Check sheet for the modelled part. Datum: model origin and axes. Units: mm. Face numbers are marked on the shaded views. A direction names the side the tool comes from. Round coordinates to 2 decimals unless told otherwise and drop trailing zeros. Write each loop counter-clockwise with the first axis right and the second up, starting at its lowest first coordinate (ties: lowest second). Pieces come first, ordered by that corner, then holes. Notation, with made-up numbers: (52, -28.75) - (100, -28.75) arc R23 cw to (100, -4.75) - close; hole circle Ø8 at (51, 10.5). An arc over 180 degrees is marked (long way). Answer as a JSON object with one key per item and string values. Group by question number.
Item 1: Thickness scan on line 1 (Z direction, x = 4.5, y = -15); line 2 (X direction, y = -6, z = -3.75); line 3 (Z direction, x = 4.25, y = -19). Record the ranges inside material, lowest first.
Item 2: Release check for a two-part mould opening along X. For the marked faces 5, 6 and 7 record: pulls with the +X half, pulls with the -X half, needs draft (parallel to the pull), parting line crosses it, or undercut.
Item 3: Gauge pin test, flat ends, axial feed: P1, Ø3, axis at y = -14.5, z = 10.5, coming from the -X side; P2, Ø4, axis at x = 8.5, y = -22, coming from the +Z side; P3, Ø2, axis at x = 2, z = 8.5, coming from the -Y side; P4, Ø0.9, axis at x = 4.5, z = 13, coming from the -Y side. Record the tip position at first contact, or that the pin passes through.
Item 4: Sectioned sample at B-B on x = 5.5. Record the boundary of the cut face in (y, z).
Item 5: Set-up check for the marked faces 1, 2, 3 and 4: record each of +Z, -Z, +X, -X, +Y, -Y from which the full face is reachable in a straight line by a thin tool's end or side.
Item 6: Sectioned sample at C-C on y = -16.5. Record the boundary of the cut face in (x, z), plus the area to 3 significant figures.
Item 7: Sectioned sample at A-A on z = 14.25. Record the boundary of the cut face in (x, y).
Item 8: Sectioned sample at D-D on x = 8.75. Record the boundary of the cut face in (y, z).
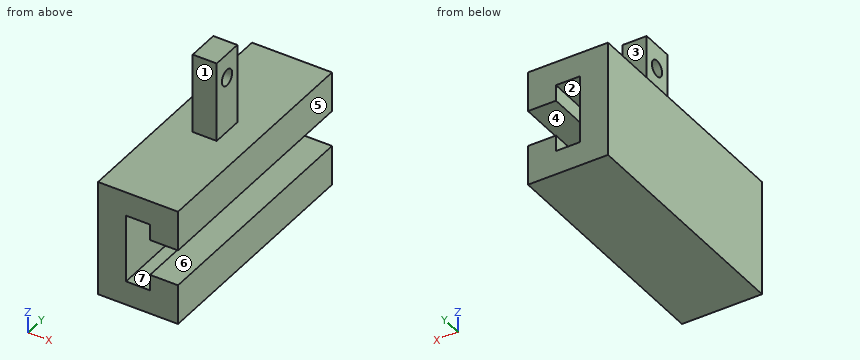
```python
from build123d import *

# Parameters (mm, degrees)
F1_DEPTH = 30
F3_DEPTH = 10
F4_R     = 1
F5_DEPTH = 5


with BuildPart() as f1:
    # F0 (on Front) → F1 (new body)
    with BuildSketch(Plane.XZ):
        Polygon((0, 7.25), (0, 0), (0, -7.25), (10, -7.25), (10, -2.25), (6.5, -2.25), (6.5, -4.25), (3.5, -4.25), (3.5, 0), (3.5, 4.25), (6.5, 4.25), (6.5, 2.25), (10, 2.25), (10, 7.25), align=None)
    extrude(amount=F1_DEPTH)

    # F2 (on face) → F3 (join)
    with BuildSketch(Plane.XY.offset(7.25)):
        Polygon((6.5, -13), (5, -13), (3.5, -13), (3.5, -15), (3.5, -17), (5, -17), (6.5, -17), (6.5, -15), align=None)
    extrude(amount=F3_DEPTH)

    # F4 (on face) → F5 (cut)
    with BuildSketch(Plane(origin=(3.5, 0, 0), x_dir=(0, -1, 0), z_dir=(-1, 0, 0))):
        with Locations((15, 14.25)):
            Circle(F4_R)
    extrude(amount=-F5_DEPTH, mode=Mode.SUBTRACT)


solid = f1.part
```
Completed:
{
 "1": {"line 1": "-7.25 to -4.25, 4.25 to 13.25, 15.25 to 17.25", "line 2": "0 to 3.5, 6.5 to 10", "line 3": "-7.25 to -4.25, 4.25 to 7.25"},
 "2": {"face 5": "pulls with the +X half", "face 6": "needs draft", "face 7": "undercut"},
 "3": {"P1": "x = 3.5", "P2": "z = 7.25", "P3": "through", "P4": "y = -17"},
 "4": {"outline": "(-30, -7.25) - (0, -7.25) - (0, -4.25) - (-30, -4.25) - close; (-30, 4.25) - (0, 4.25) - (0, 7.25) - (-13, 7.25) - (-13, 17.25) - (-17, 17.25) - (-17, 7.25) - (-30, 7.25) - close; hole circle Ø2 at (-15, 14.25)"},
 "5": {"face 1": "+Z, +X, -X, -Y", "face 2": "+Y, -Y", "face 3": "+Z, +X, -X, +Y", "face 4": "+X, +Y, -Y"},
 "6": {"outline": "(0, -7.25) - (10, -7.25) - (10, -2.25) - (6.5, -2.25) - (6.5, -4.25) - (3.5, -4.25) - (3.5, 4.25) - (6.5, 4.25) - (6.5, 2.25) - (10, 2.25) - (10, 7.25) - (6.5, 7.25) - (6.5, 17.25) - (3.5, 17.25) - (3.5, 7.25) - (0, 7.25) - close", "area": "134 mm²"},
 "7": {"outline": "(3.5, -17) - (6.5, -17) - (6.5, -16) - (3.5, -16) - close; (3.5, -14) - (6.5, -14) - (6.5, -13) - (3.5, -13) - close"},
 "8": {"outline": "(-30, -7.25) - (0, -7.25) - (0, -2.25) - (-30, -2.25) - close; (-30, 2.25) - (0, 2.25) - (0, 7.25) - (-30, 7.25) - close"}
}
